Work out the finished part from the listing and answer in its coordinate system (mm). Give positions to 0.01 mm unless a question says otherwise; leave off trailing zeros. Order: outer loops, then holes, each group sorted by start corner. A loop starts at its lowest first (then second) coordinate and runs counter-clockwise, first axis right, second up. Notation, with made-up numbers: (-32, -1.75) -> (-25, -1.75) arc R26 ccw to (-25, 37.25) -> close; hole circle Ø2 at (19, 82). An arc over 180 degrees is marked (long way). Use a Markdown table: item, result. Add a question column.
Autodesk Inventor part; units mm, degrees
ref_plane "Work Plane1" through (0, 101.6, 0) normal (0, 1, 0) x (1, 0, 0)
ref_plane "YZ Plane" through (0, 0, 0) normal (1, 0, 0) x (0, 1, 0)
ref_plane "XZ Plane" through (0, 0, 0) normal (0, 1, 0) x (-1, 0, 0)
sketch "Sketch1" plane through (0, 0, 0) normal (0, 1, 0) x (-1, 0, 0)
  line L0 (0, 0) -> (25.4, 0)
  line L1 (25.4, 0) -> (25.4, -25.4)
  line L2 (25.4, -25.4) -> (0, -25.4)
  line L3 (0, -25.4) -> (0, 0)
  dimension "d0" = 25.4
  dimension "d1" = 25.4
extrude "Extrusion1" add sketch "Sketch1" along normal blind 203.2
hole "Hole1" at (-12.7, 190.5, 0) direction (0, 0, -1) diameter 6.35 end through all
ref_plane "Work Plane1" through (0, 101.6, 0) normal (0, 1, 0) x (1, 0, 0)
mirror "Mirror1" about plane through (0, 101.6, 0) normal (0, 1, 0) of "Hole1"
fillet "Fillet1" radius 12.7 4 edges at (0, 203.2, -12.7) (-25.4, 203.2, -12.7) (0, 0, -12.7) (-25.4, 0, -12.7)
chamfer "Chamfer1" distance 2.54 angle 45 8 edges at (0, 101.6, 0) (-3.7197, 199.4803, 0) (-25.4, 101.6, 0) (-3.7197, 3.7197, 0) (0, 101.6, -25.4) (-3.7197, 199.4803, -25.4) (-25.4, 101.6, -25.4) (-3.7197, 3.7197, -25.4)
properties part number "shortBar"
1) A flat-ended cylindrical pin translates along its axis: pin 1 (6 mm diameter, centred on x = -5, z = -2.5, fed in from -Y). Find the tip coordinate at first contact, or state that the pin passes through.
2) The part is cut by section B-B, the plane y = 132.5. Determine the outline of the cut face in (x, z), then the cut area to 3 significant figures.
3) Straight lines are drawn through the part: line 1 (Y direction, x = -12.7, z = -8.25) (3 decimals); line 2 (Y direction, x = -10.5, z = -22); line 3 (X direction, y = 190.5, z = -10) (3 decimals). For each, find the intervals that lie inside material, in ascending order.
4) The part is cut by section A-A, the plane z = -10.5. State how many separate pieces and enclosed holes the cut face has, then the cut area to 3 significant figures.
5) Determine the mould class of faces 1 (the conical face through (-20.311, 4.92, -0.723)), 2 (the cylindrical face through (-12.84, 193.67, -12.88)), 3 (the flat face through (0, 100, -13)) for opening direction Y: released by +Y, released by -Y, zero draft, split by the parting line, or undercut.
A:
| question | item | result |
|---|---|---|
| 1 | pin 1 | y = 0.9 |
| 2 | outline | (-25.4, -22.86) -> (-22.86, -25.4) -> (-2.54, -25.4) -> (0, -22.86) -> (0, -2.54) -> (-2.54, 0) -> (-22.86, 0) -> (-25.4, -2.54) -> close |
| 2 | area | 632 mm^2 |
| 3 | line 1 | 0 to 9.525, 15.875 to 187.325, 193.675 to 203.2 |
| 3 | line 2 | 0.19 to 10.41, 14.99 to 188.21, 192.79 to 203.01 |
| 3 | line 3 | -25.4 to -15.875, -9.525 to 0 |
| 4 | separate pieces | 1 |
| 4 | enclosed holes | 2 |
| 4 | area | 4,960 mm^2 |
| 5 | face 1 | released by -Y |
| 5 | face 2 | undercut |
| 5 | face 3 | zero draft |
